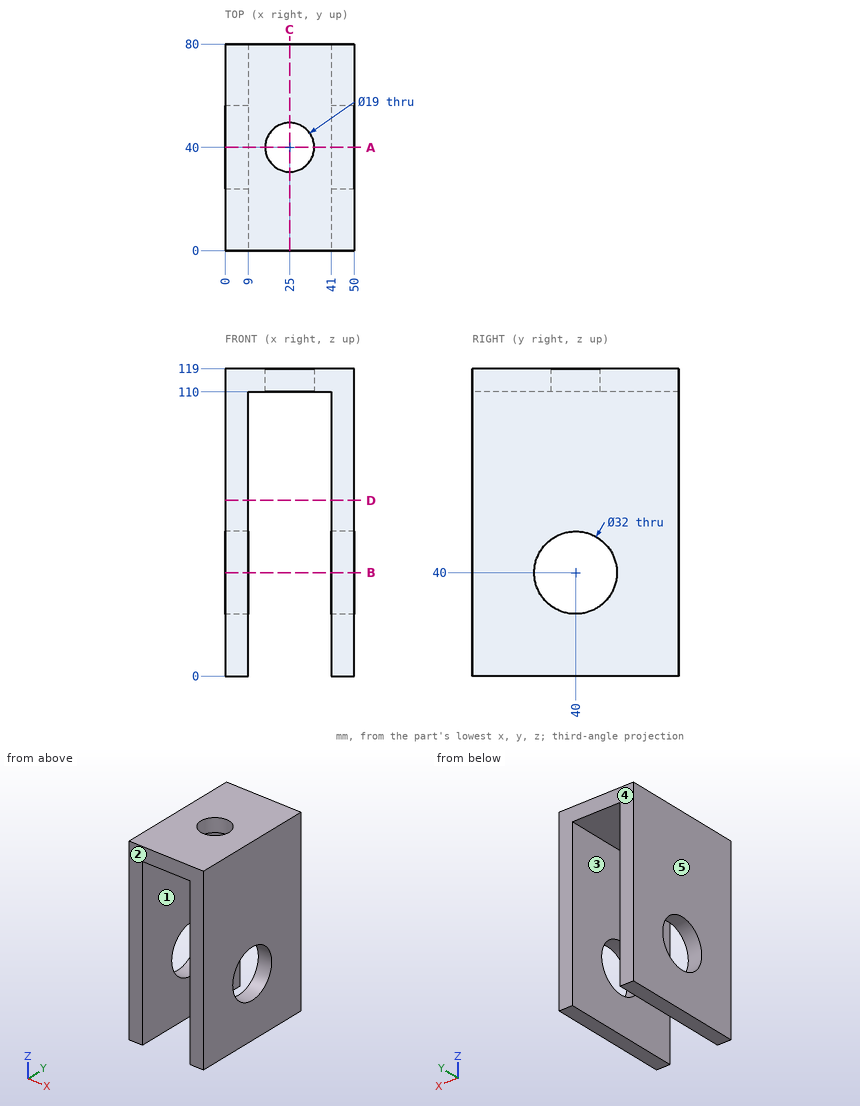
Part print with two shaded views. Sizes in mm from the minimum x, y, z corner. A direction names the side the tool comes from. Give positions to 0.01 mm unless a question says otherwise; leave off trailing zeros. Order: outer loops, then holes, each group sorted by start corner. A loop starts at its lowest first (then second) coordinate and runs counter-clockwise, first axis right, second up.
1) Saw through at A-A, the plane y = 40. Write the cut outline in (x, z).
2) Pin check, flat tips, straight feed: pin 1 (6 mm diameter, centred on y = 18.5, z = 37, fed in from -X); pin 2 (8 mm diameter, centred on x = 18.5, y = 68, fed in from -Z); pin 3 (5 mm diameter, centred on y = 33, z = 51, fed in from -X). Stop position of each tip, or through.
3) 3-axis set-ups, long thin cutter, end or side, ignore diameter. For the marked faces 1 and 2: which of +Z, -Z, +X, -X, +Y, -Y reach the whole face in a straight line?
4) Saw through at B-B, the plane z = 40. Write the cut outline in (x, y), then the cut area to 3 significant figures.
5) Saw through at C-C, the plane x = 25. Write the cut outline in (y, z).
6) Saw through at D-D, the plane z = 68. Write the cut outline in (x, y).
7) Wall check: probe 1 along X at (y, z) = (48.5, 86); probe 2 along Y at (x, z) = (25, 113); probe 3 along Z at (x, y) = (43, 40). Give the ranges that are in metal, low to high.
8) Mould opens along X. For the marked faces 3, 4 and 5 say: +X half, -X half, draft (parallel to the pull), parting line (faces both ways), or undercut.
Computed:
1. outline: (0, 0) - (9, 0) - (9, 24) - (0, 24) - close; (0, 56) - (9, 56) - (9, 110) - (15.5, 110) - (15.5, 119) - (0, 119) - close; (34.5, 110) - (41, 110) - (41, 56) - (50, 56) - (50, 119) - (34.5, 119) - close; (41, 0) - (50, 0) - (50, 24) - (41, 24) - close
2. pin 1: stops at x = 0
2. pin 2: stops at z = 110
2. pin 3: passes through
3. face 1: -Z, +Y, -Y
3. face 2: +Z, -Z, +X, -X, -Y
4. outline: (0, 0) - (9, 0) - (9, 24) - (0, 24) - close; (0, 56) - (9, 56) - (9, 80) - (0, 80) - close; (41, 0) - (50, 0) - (50, 24) - (41, 24) - close; (41, 56) - (50, 56) - (50, 80) - (41, 80) - close
4. area: 864 mm2
5. outline: (0, 110) - (30.5, 110) - (30.5, 119) - (0, 119) - close; (49.5, 110) - (80, 110) - (80, 119) - (49.5, 119) - close
6. outline: (0, 0) - (9, 0) - (9, 80) - (0, 80) - close; (41, 0) - (50, 0) - (50, 80) - (41, 80) - close
7. probe 1: x = 0 to 9, 41 to 50
7. probe 2: y = 0 to 30.5, 49.5 to 80
7. probe 3: z = 0 to 24, 56 to 119
8. face 3: undercut
8. face 4: draft
8. face 5: -X half
